from build123d import *

# Parameters (mm, degrees)
SKETCH1_W               = 81.6
SKETCH1_H               = 0.9
SKETCH1_H_2             = 7.4
BOSS_EXTRUDE1_DEPTH     = 9.8
SKETCH5_W               = 9.8
SKETCH5_H               = 9.2
CUT_EXTRUDE3_DEPTH      = 1.5
CUT_EXTRUDE1_REACH      = 84.315
CUT_EXTRUDE1_END_RADIUS = 3.25
SKETCH3_R               = 1.45
CUT_EXTRUDE2_REACH      = 84.315
CUT_EXTRUDE2_END_RADIUS = 11.25
SKETCH4_R               = 2


with BuildPart() as part:
    # Sketch1 → Boss-Extrude1 (new body)
    # profile 1 of 3: a face of its own
    with BuildSketch(Plane(origin=(0, 0, 0), x_dir=(0, 0, -1), z_dir=(1, 0, 0))):
        with Locations((0, 4.15)):
            Rectangle(SKETCH1_W, SKETCH1_H)
    # profile 2 of 3: a face of its own
    with BuildSketch(Plane(origin=(0, 0, 0), x_dir=(0, 0, -1), z_dir=(1, 0, 0))):
        Rectangle(SKETCH1_W, SKETCH1_H_2)
        with BuildLine():
            ThreePointArc((-2.25, -3.45), (-5.5, -0.2), (-2.25, 3.05))
            Line((-2.25, 3.05), (2.25, 3.05))
            ThreePointArc((2.25, 3.05), (5.5, -0.2), (2.25, -3.45))
            Line((2.25, -3.45), (-2.25, -3.45))
        make_face(mode=Mode.SUBTRACT)
    # profile 3 of 3: a face of its own
    with BuildSketch(Plane(origin=(0, 0, 0), x_dir=(0, 0, -1), z_dir=(1, 0, 0))):
        with Locations((0, -4.15)):
            Rectangle(SKETCH1_W, SKETCH1_H)
    extrude(amount=BOSS_EXTRUDE1_DEPTH)

    # Sketch5 → Cut-Extrude3 (cut)
    with BuildSketch(Plane.XY.offset(40.8)):
        with Locations((4.9, 0)):
            Rectangle(SKETCH5_W, SKETCH5_H)
        with BuildLine():
            Line((7, 2.5), (0, 2.5))
            Line((0, 2.5), (0, -2.5))
            Line((0, -2.5), (7, -2.5))
            ThreePointArc((7, -2.5), (7.707106781, -2.207106781), (8, -1.5))
            Line((8, -1.5), (8, 1.5))
            ThreePointArc((8, 1.5), (7.707106781, 2.207106781), (7, 2.5))
        make_face(mode=Mode.SUBTRACT)
    cut_extrude3 = extrude(amount=-CUT_EXTRUDE3_DEPTH, mode=Mode.SUBTRACT)

    # Cut-Extrude1: up to this cylinder (the profile starts outside it)
    cut_extrude1_end = Plane(origin=(4.9, -0.2, 2.25), z_dir=(-1, 0, 0)) * Cylinder(CUT_EXTRUDE1_END_RADIUS, 176.13, mode=Mode.PRIVATE)
    # Sketch3 → Cut-Extrude1 (cut, up to the surface)
    with BuildSketch(Plane.XY.offset(40.8), mode=Mode.PRIVATE) as cut_extrude1_sk1:
        with Locations((4.9, 0)):
            Circle(SKETCH3_R)
    cut_extrude1_tool1 = extrude(cut_extrude1_sk1.sketch, amount=-CUT_EXTRUDE1_REACH, mode=Mode.PRIVATE) - cut_extrude1_end
    cut_extrude1 = cut_extrude1_tool1.solids().sort_by_distance((4.9, 0, 40.8))[0]
    add(cut_extrude1, mode=Mode.SUBTRACT)

    # Cut-Extrude2: up to this cylinder (the profile starts outside it)
    cut_extrude2_end = Plane(origin=(4.9, -0.2, 2.25), z_dir=(-1, 0, 0)) * Cylinder(CUT_EXTRUDE2_END_RADIUS, 192.13, mode=Mode.PRIVATE)
    # Sketch4 → Cut-Extrude2 (cut, up to the surface)
    with BuildSketch(Plane.XY.offset(40.8), mode=Mode.PRIVATE) as cut_extrude2_sk1:
        with Locations((4.9, 0)):
            Circle(SKETCH4_R)
    cut_extrude2_tool1 = extrude(cut_extrude2_sk1.sketch, amount=-CUT_EXTRUDE2_REACH, mode=Mode.PRIVATE) - cut_extrude2_end
    cut_extrude2 = cut_extrude2_tool1.solids().sort_by_distance((4.9, 0, 40.8))[0]
    add(cut_extrude2, mode=Mode.SUBTRACT)

    # Mirror5: Cut-Extrude3, Cut-Extrude1, Cut-Extrude2 across plane
    add(cut_extrude3.mirror(Plane.XY), mode=Mode.SUBTRACT)
    add(cut_extrude1.mirror(Plane.XY), mode=Mode.SUBTRACT)
    add(cut_extrude2.mirror(Plane.XY), mode=Mode.SUBTRACT)


solid = part.part
Build history of the part. All positions in model axes, mm. A direction names the side the tool comes from. Give positions to 0.01 mm unless a question says otherwise; leave off trailing zeros. Loops run counter-clockwise (first coordinate to the right, second up) from the corner with the lowest first, then second, coordinate; pieces in that order, holes last. Notation, with made-up numbers: (84.5, -28.5) -> (112.5, -28.5) arc R17 ccw to (112.5, -10.5) -> close; hole circle Ø8 at (17.5, 35). An arc over 180 degrees is marked (long way). Answer in a Markdown table with one row per item.
Item 1: Mould opens along X. For faces 1 (the flat face through (3.06, -1.15, -40.8)), 2 (the cylindrical face through (6.28, 0.44, -9.33)), 3 (the cylindrical face through (3.3, -1.2, -27.2)), 4 (the flat face through (9.8, 4, 1)) say: pulls with the +X half, pulls with the -X half, needs draft (parallel to the pull), parting line crosses it, or undercut.
Findings below:
| item | result |
|---|---|
| face 1 | needs draft |
| face 2 | undercut |
| face 3 | undercut |
| face 4 | pulls with the +X half |
Item 2: Probe line 1 along Y through (x, z) = (4.9, -33.25); line 2 along Y through (x, z) = (4.9, 8); line 3 along Z through (x, y) = (2, 2.75). List the from-to ranges inside material, lowest first. Write a range as [from, to].
Findings below:
| item | result |
|---|---|
| line 1 | y = [-4.6, -2], [2, 4.6] |
| line 2 | y = [-4.6, -1.45], [1.45, 4.6] |
| line 3 | z = [-39.3, -3.61], [3.61, 39.3] |
Item 3: Flat gauge pins, fed straight in: P1, Ø0.8, axis at x = 5, z = 40.5, coming from the -Y side; P2, Ø3, axis at x = 4.9, y = 0, coming from the +Z side; P3, Ø2, axis at y = 2, z = -1, coming from the +X side. Where does each tip first touch, or does it go through?
Findings below:
| item | result |
|---|---|
| P1 | stops at y = -2.5 |
| P2 | stops at z = 13.5 |
| P3 | passes through |
Item 4: Slice it at A-A on z = 0. Write the cut outline in (x, y), plus the area to 3 significant figures.
Findings below:
| item | result |
|---|---|
| outline | (0, -4.6) -> (9.8, -4.6) -> (9.8, -3.45) -> (0, -3.45) -> close; (0, 3.05) -> (9.8, 3.05) -> (9.8, 4.6) -> (0, 4.6) -> close |
| area | 26.5 mm² |
Item 5: Slice it at D-D on x = 8.75. Write the cut outline in (y, z).
Findings below:
| item | result |
|---|---|
| outline | (-4.6, -39.3) -> (4.6, -39.3) -> (4.6, 39.3) -> (-4.6, 39.3) -> close; hole (-3.45, -2.25) arc R3.25 ccw to (3.05, -2.25) -> (3.05, 2.25) arc R3.25 ccw to (-3.45, 2.25) -> close |
Item 6: Slice it at C-C on y = 0. Write the cut outline in (x, z).
Findings below:
| item | result |
|---|---|
| outline | (0, -40.8) -> (2.9, -40.8) -> (2.9, -13.5) -> (3.45, -13.5) -> (3.45, -5.49) -> (0, -5.49) -> close; (0, 5.49) -> (3.45, 5.49) -> (3.45, 13.5) -> (2.9, 13.5) -> (2.9, 40.8) -> (0, 40.8) -> close; (6.35, -13.5) -> (6.9, -13.5) -> (6.9, -40.8) -> (8, -40.8) -> (8, -39.3) -> (9.8, -39.3) -> (9.8, -5.49) -> (6.35, -5.49) -> close; (6.35, 5.49) -> (9.8, 5.49) -> (9.8, 39.3) -> (8, 39.3) -> (8, 40.8) -> (6.9, 40.8) -> (6.9, 13.5) -> (6.35, 13.5) -> close |
Item 7: Tool access for faces 5 (the cylindrical face through (3.74, -1.24, -5.33)), 6 (the flat face through (6, 3, 39.3)), 7 (the flat face through (4, 2.5, -40)): list every direction of +Z, -Z, +X, -X, +Y, -Y with a clear straight run to the whole face (end or side of a thin tool).
Findings below:
| item | result |
|---|---|
| face 5 | +X, -X |
| face 6 | +Z, +X |
| face 7 | -Z, +X, -X, +Y |
